```python
from build123d import *
from build123d.topology import SkipClean

# Parameters (mm, degrees)
SKETCH_1_R               = 2.35
SKETCH_1_R_2             = 8.9
EXTRUDE_1_DEPTH          = 5
EXTRUDE_2_DEPTH          = 44.5
EXTRUDE_2_DEPTH_BACK     = 5
EXTRUDE_START            = -9
EXTRUDE_3_DEPTH          = 9
SKETCH_5_R               = 1.8
CUT_EXTRUDE_2_DEPTH      = 19
CUT_EXTRUDE_5_DEPTH      = 10
CUT_EXTRUDE_5_DEPTH_BACK = 10
SKETCH_9_W               = 118.709111843
SKETCH_9_H               = 68.105929764
SKETCH_9_W_2             = 50.6
SKETCH_9_H_2             = 49.5
SKETCH_10_W              = 50.6
SKETCH_10_H              = 4.95
CUT_EXTRUDE_6_DEPTH      = 67.841008738
SKETCH_11_R              = 2.3
CUT_EXTRUDE_7_DEPTH      = 67.841008738
SKETCH_12_R              = 2.3
CUT_EXTRUDE_8_DEPTH      = 10
SKETCH_13_R              = 4.5
CUT_EXTRUDE_9_DEPTH      = 2
SKETCH_14_R              = 1.7
EXTRUDE_4_DEPTH          = 4


with BuildPart() as part:
    # Sketch 1 → Extrude 1 (new body)
    with BuildSketch(Plane.XY):
        with BuildLine():
            ThreePointArc((-13.750457514, -22.60807726), (-15.630598029, -22.207924557), (-17.367665677, -23.031117444))
            ThreePointArc((-17.367665677, -23.031117444), (-24.500349004, -22.846945062), (-24.186521915, -15.718789377))
            ThreePointArc((-24.186521915, -15.718789377), (-23.24416257, -14.043376172), (-23.512188549, -12.139902343))
            ThreePointArc((-23.512188549, -12.139902343), (-26.460924905, -0.14032965), (-23.639624978, 11.889843151))
            ThreePointArc((-23.639624978, 11.889843151), (-23.371598999, 13.79331698), (-24.313958344, 15.468730186))
            ThreePointArc((-24.313958344, 15.468730186), (-24.723627875, 23.005643376), (-17.178817704, 23.226389957))
            ThreePointArc((-17.178817704, 23.226389957), (-15.441750056, 22.403197069), (-13.561609541, 22.803349773))
            ThreePointArc((-13.561609541, 22.803349773), (-0.542505729, 26.377270873), (12.476598084, 22.803349773))
            ThreePointArc((12.476598084, 22.803349773), (14.356738599, 22.403197069), (16.093806247, 23.226389957))
            ThreePointArc((16.093806247, 23.226389957), (25.011719512, 23.858129918), (24.906055495, 14.918493041))
            ThreePointArc((24.906055495, 14.918493041), (24.067269609, 13.359986921), (24.253003064, 11.599871535))
            ThreePointArc((24.253003064, 11.599871535), (26.972168217, 0.141967553), (24.253003064, -11.31593643))
            ThreePointArc((24.253003064, -11.31593643), (23.984977085, -13.219410259), (24.92733643, -14.894823465))
            ThreePointArc((24.92733643, -14.894823465), (24.934120683, -23.972974271), (15.904958274, -23.031117444))
            ThreePointArc((15.904958274, -23.031117444), (14.167890626, -22.207924557), (12.287750111, -22.60807726))
            ThreePointArc((12.287750111, -22.60807726), (-0.731353702, -26.18199836), (-13.750457514, -22.60807726))
        make_face()
        with Locations((-14.5, 0)):
            Circle(SKETCH_1_R, mode=Mode.SUBTRACT)
        with Locations((14.5, 0)):
            Circle(SKETCH_1_R, mode=Mode.SUBTRACT)
        Circle(SKETCH_1_R_2, mode=Mode.SUBTRACT)
    extrude(amount=EXTRUDE_1_DEPTH)

    # Sketch 2 → Extrude 2 (add, two sides: drawn at the far end of the back side and taken through both)
    with BuildSketch(Plane.XY.offset(5).offset(-EXTRUDE_2_DEPTH_BACK)):
        with BuildLine():
            Line((-25.3, 0), (-21.3, 0))
            ThreePointArc((-21.3, 0), (0, -21.3), (21.3, 0))
            Line((21.3, 0), (25.3, 0))
            Line((25.3, 0), (25.3, -13.25))
            ThreePointArc((25.3, -13.25), (28.228932188, -20.321067812), (35.3, -23.25))
            Line((35.3, -23.25), (50, -23.25))
            Line((50, -23.25), (50, -28.25))
            Line((50, -28.25), (-50, -28.25))
            Line((-50, -28.25), (-50, -23.25))
            Line((-50, -23.25), (-35.3, -23.25))
            ThreePointArc((-35.3, -23.25), (-28.228932188, -20.321067812), (-25.3, -13.25))
            Line((-25.3, -13.25), (-25.3, 0))
        make_face()
    extrude(amount=EXTRUDE_2_DEPTH + EXTRUDE_2_DEPTH_BACK)

    # Sketch 4 → Extrude 3 (add)
    with SkipClean():  # the faces are left unmerged after this step: merging them gives an invalid solid
        with BuildSketch(Plane.XY.offset(49.5).offset(EXTRUDE_START)):
            with BuildLine():
                Line((21.3, 0), (25.3, 0))
                ThreePointArc((25.3, 0), (20.373090978, 18.07450089), (5.5, 29.465426213))
                Line((5.5, 29.465426213), (5.5, 35.916188423))
                Line((5.5, 35.916188423), (1.5, 35.916188423))
                Line((1.5, 35.916188423), (1.5, 29.916188423))
                Line((1.5, 29.916188423), (1.5, 21.247117452))
                ThreePointArc((1.5, 21.247117452), (15.582682696, 14.521363572), (21.3, 0))
            make_face()
            with BuildLine():
                Line((-25.3, 0), (-21.3, 0))
                ThreePointArc((-21.3, 0), (-15.582682696, 14.521363572), (-1.5, 21.247117452))
                Line((-1.5, 21.247117452), (-1.5, 29.916188423))
                Line((-1.5, 29.916188423), (-1.5, 35.916188423))
                Line((-1.5, 35.916188423), (-5.5, 35.916188423))
                Line((-5.5, 35.916188423), (-5.5, 29.465426213))
                ThreePointArc((-5.5, 29.465426213), (-20.373090978, 18.07450089), (-25.3, 0))
            make_face()
        extrude(amount=EXTRUDE_3_DEPTH)

    # Sketch 5 → Cut-Extrude 2 (cut)
    with SkipClean():  # the faces are left unmerged after this step: merging them gives an invalid solid
        with BuildSketch(Plane.ZY.offset(5.5)):
            with Locations(Location((45, 32.690807318, 0), (0, 0, 270))):
                Circle(SKETCH_5_R)
        extrude(amount=-CUT_EXTRUDE_2_DEPTH, mode=Mode.SUBTRACT)

    # Sketch 9 → Cut-Extrude 5 (cut, two sides: drawn at the far end of the back side and taken through both)
    with SkipClean():  # the faces are left unmerged after this step: merging them gives an invalid solid
        with BuildSketch(Plane(origin=(0, -23.25, 0), x_dir=(1, 0, 0), z_dir=(0, 1, 0)).offset(-CUT_EXTRUDE_5_DEPTH_BACK)):
            with Locations((-0.535798399, -23.678403203)):
                Rectangle(SKETCH_9_W, SKETCH_9_H)
            with Locations((0, -24.75)):
                Rectangle(SKETCH_9_W_2, SKETCH_9_H_2, mode=Mode.SUBTRACT)
        extrude(amount=CUT_EXTRUDE_5_DEPTH + CUT_EXTRUDE_5_DEPTH_BACK, mode=Mode.SUBTRACT)

    # Sketch 10 → Cut-Extrude 6 (cut, through all)
    with SkipClean():  # the faces are left unmerged after this step: merging them gives an invalid solid
        with BuildSketch(Plane.XY.offset(49.5)):
            with Locations((0, -25.775)):
                Rectangle(SKETCH_10_W, SKETCH_10_H)
        extrude(amount=-CUT_EXTRUDE_6_DEPTH, mode=Mode.SUBTRACT)

    # Sketch 11 → Cut-Extrude 7 (cut, through all)
    with SkipClean():  # the faces are left unmerged after this step: merging them gives an invalid solid
        with BuildSketch(Plane(origin=(0, 0, 0), x_dir=(-1, 0, 0), z_dir=(0, 0, -1))):
            with Locations((-20.843580496, -19.436953262)):
                Circle(SKETCH_11_R)
            with Locations((20.843580496, -19.436953262)):
                Circle(SKETCH_11_R)
        extrude(amount=-CUT_EXTRUDE_7_DEPTH, mode=Mode.SUBTRACT)

    # Sketch 12 → Cut-Extrude 8 (cut)
    with SkipClean():  # the faces are left unmerged after this step: merging them gives an invalid solid
        with BuildSketch(Plane(origin=(0, 0, 0), x_dir=(-1, 0, 0), z_dir=(0, 0, -1))):
            with Locations((-20.843580496, 19.436953262)):
                Circle(SKETCH_12_R)
            with Locations((20.843580496, 19.436953262)):
                Circle(SKETCH_12_R)
        extrude(amount=-CUT_EXTRUDE_8_DEPTH, mode=Mode.SUBTRACT)

    # Sketch 13 → Cut-Extrude 9 (cut)
    with SkipClean():  # the faces are left unmerged after this step: merging them gives an invalid solid
        with BuildSketch(Plane(origin=(0, 0, 0), x_dir=(-1, 0, 0), z_dir=(0, 0, -1))):
            with Locations((-14.5, 0)):
                Circle(SKETCH_13_R)
            with Locations((14.5, 0)):
                Circle(SKETCH_13_R)
        extrude(amount=-CUT_EXTRUDE_9_DEPTH, mode=Mode.SUBTRACT)

    # Sketch 14 → Extrude 4 (add)
    # profile 1 of 4: a face of its own
    with SkipClean():  # the faces are left unmerged after this step: merging them gives an invalid solid
        with BuildSketch(Plane.XZ.offset(23.3)):
            with BuildLine():
                Line((-30, 39.7), (-25.3, 39.7))
                Line((-25.3, 39.7), (-25.3, 30.3))
                Line((-25.3, 30.3), (-30, 30.3))
                ThreePointArc((-30, 30.3), (-34.7, 35), (-30, 39.7))
            make_face()
            with Locations(Location((-30, 35, 0), (0, 0, 270))):
                Circle(SKETCH_14_R, mode=Mode.SUBTRACT)
        # profile 2 of 4: a face of its own
        with BuildSketch(Plane.XZ.offset(23.3)):
            with BuildLine():
                Line((25.3, 39.7), (25.3, 30.3))
                Line((25.3, 30.3), (30, 30.3))
                ThreePointArc((30, 30.3), (34.7, 35), (30, 39.7))
                Line((30, 39.7), (25.3, 39.7))
            make_face()
            with Locations(Location((30, 35, 0), (0, 0, 90))):
                Circle(SKETCH_14_R, mode=Mode.SUBTRACT)
        # profile 3 of 4: a face of its own
        with BuildSketch(Plane.XZ.offset(23.3)):
            with BuildLine():
                Line((30, 0.3), (25.3, 0.3))
                Line((25.3, 0.3), (25.3, 9.7))
                Line((25.3, 9.7), (30, 9.7))
                ThreePointArc((30, 9.7), (34.7, 5), (30, 0.3))
            make_face()
            with Locations(Location((30, 5, 0), (0, 0, 270))):
                Circle(SKETCH_14_R, mode=Mode.SUBTRACT)
        # profile 4 of 4: a face of its own
        with BuildSketch(Plane.XZ.offset(23.3)):
            with BuildLine():
                Line((-25.3, 0.3), (-25.3, 9.7))
                Line((-25.3, 9.7), (-30, 9.7))
                ThreePointArc((-30, 9.7), (-34.7, 5), (-30, 0.3))
                Line((-30, 0.3), (-25.3, 0.3))
            make_face()
            with Locations(Location((-30, 5, 0), (0, 0, 90))):
                Circle(SKETCH_14_R, mode=Mode.SUBTRACT)
        extrude(amount=-EXTRUDE_4_DEPTH)


solid = part.part
```
Build history of the part. All positions in model axes, mm. A direction names the side the tool comes from. Give positions to 0.01 mm unless a question says otherwise; leave off trailing zeros. Loops run counter-clockwise (first coordinate to the right, second up) from the corner with the lowest first, then second, coordinate; pieces in that order, holes last. Notation, with made-up numbers: (7, 62.25) - (59, 62.25) arc R11 cw to (59, 77.25) - close; hole circle Ø7 at (7.25, 25.5). An arc over 180 degrees is marked (long way). Use a Markdown table: item, result.
(1) Which spindle directions (+Z, -Z, +X, -X, +Y, -Y) get a long thin tool onto all of the face, cutting with end or side? Do faces 5 (the face through (-0.734, 26.377, 2.465)), 6 (the face through (-5, 8, 5)), 7 (the face through (13, 19, 40.5)), 8 (the face through (28, -21, 9.7)). Say none if no direction does.
Taken from the geometry:
| item | result |
|---|---|
| face 5 | -Z, +Y |
| face 6 | +Y |
| face 7 | +X, -X, +Y |
| face 8 | +X, +Y, -Y |
(2) Band-saw the part on B-B (x = 15). Give the cut face in (y, z), and give its area (3 significant figures).
Taken from the geometry:
| item | result |
|---|---|
| outline | (-23.3, 0) - (-4.47, 0) - (-4.47, 2) - (-2.3, 2) - (-2.3, 5) - (-15.12, 5) - (-15.12, 49.5) - (-23.3, 49.5) - close; (2.3, 2) - (4.47, 2) - (4.47, 0) - (22.55, 0) - (22.55, 5) - (2.3, 5) - close; (15.12, 40.5) - (24.08, 40.5) - (24.08, 49.5) - (15.12, 49.5) - close |
| area | 642 mm2 |
(3) Band-saw the part on C-C (z = 12.5). Give the cut face in (x, y).
Taken from the geometry:
| item | result |
|---|---|
| outline | (-25.3, -23.3) - (25.3, -23.3) - (25.3, 0) - (21.3, 0) arc R21.3 cw to (-21.3, 0) - (-25.3, 0) - close; hole circle Ø4.6 at (-20.84, -19.44); hole circle Ø4.6 at (20.84, -19.44) |
(4) Wall check: line 1 along X through (y, z) = (-22.2, 35); line 2 along X through (y, z) = (19.5, 2); line 3 along Z through (x, y) = (27.5, -20). Give the ranges that are in metal, low to high.
Taken from the geometry:
| item | result |
|---|---|
| line 1 | -34.7 to -31.7, -28.3 to 28.3, 31.7 to 34.7 |
| line 2 | -26.11 to -23.14, -18.54 to 18.54, 23.14 to 26.92 |
| line 3 | 0.3 to 9.7, 30.3 to 39.7 |
(5) Band-saw the part on A-A (z = 35). Give the cut face in (x, y).
Taken from the geometry:
| item | result |
|---|---|
| outline | (-34.7, -23.3) - (-31.7, -23.3) - (-31.7, -19.3) - (-34.7, -19.3) - close; (-28.3, -23.3) - (28.3, -23.3) - (28.3, -19.3) - (25.3, -19.3) - (25.3, 0) - (21.3, 0) arc R21.3 cw to (-21.3, 0) - (-25.3, 0) - (-25.3, -19.3) - (-28.3, -19.3) - close; (31.7, -23.3) - (34.7, -23.3) - (34.7, -19.3) - (31.7, -19.3) - close; hole circle Ø4.6 at (-20.84, -19.44); hole circle Ø4.6 at (20.84, -19.44) |
(6) Band-saw the part on D-D (x = 0). Give the cut face in (y, z).
Taken from the geometry:
| item | result |
|---|---|
| outline | (-23.3, 0) - (-8.9, 0) - (-8.9, 5) - (-21.3, 5) - (-21.3, 49.5) - (-23.3, 49.5) - close; (8.9, 0) - (26.37, 0) - (26.37, 5) - (8.9, 5) - close |
(7) Pull direction Y, two halves, no side cores. Call faces 1 (the face through (23, 0, 23)), 2 (the face through (-16.848, 0.103, 3.479)), 3 (the face through (-13, 19, 40.5)), 4 (the face through (19, 0, 1)): +Y half, -Y half, draft (parallel to the pull), parting line (faces both ways), or undercut.
Taken from the geometry:
| item | result |
|---|---|
| face 1 | +Y half |
| face 2 | undercut |
| face 3 | draft |
| face 4 | undercut |
(8) Drop flat-ended pins along their axis: pin 1 Ø5 at (y, z) = (19.5, 43) entering from -X; pin 2 Ø1.2 at (x, z) = (24, 17) entering from +Y; pin 3 Ø4.5 at (y, z) = (26.5, 45) entering from +X. Give the stop position or say it passes through.
Taken from the geometry:
| item | result |
|---|---|
| pin 1 | x = -21.06 |
| pin 2 | y = 0 |
| pin 3 | x = 14.8 |
